from build123d import *

# Parameters (mm, degrees)
SKETCH2_R           = 2.35
BOSS_EXTRUDE1_DEPTH = 1.85
SKETCH3_R           = 2.35
BOSS_EXTRUDE2_DEPTH = 0.65
BOSS_EXTRUDE2_DRAFT = -45
SKETCH4_R           = 3
BOSS_EXTRUDE3_DEPTH = 6.5
CUT_EXTRUDE1_DEPTH  = 3
CHAMFER1_SIZE       = 0.6135


with BuildPart() as part:
    # Sketch1 → Revolve1 (revolve)
    with BuildSketch(Plane.XY, mode=Mode.PRIVATE) as revolve1_sk:
        with BuildLine():
            Line((-6, 6.5), (-6, 0))
            Line((-6, 0), (100, 0))
            Line((100, 0), (100, 4))
            Line((100, 4), (1, 4))
            Line((1, 4), (0.7, 3.7))
            ThreePointArc((0.7, 3.7), (0.201222236, 3.864777793), (0, 4.35))
            Line((0, 4.35), (0, 6.5))
            Line((0, 6.5), (-6, 6.5))
        make_face()
    revolve(revolve1_sk.sketch.rotate(Axis((-6, 0, 0), (1, 0, 0)), 270), axis=Axis((-6, 0, 0), (1, 0, 0)))

    # Sketch2 → Boss-Extrude1 (add)
    with BuildSketch(Plane(origin=(100, 0, 0), x_dir=(0, 0, -1), z_dir=(1, 0, 0))):
        with Locations(Location((0, 0, 0), (0, 0, 180))):
            Circle(SKETCH2_R)
    extrude(amount=BOSS_EXTRUDE1_DEPTH)


with BuildPart() as boss_extrude2_tool:
    # Sketch3 → Boss-Extrude2 (with draft: the straight prism first)
    with BuildSketch(Plane(origin=(101.85, 0, 0), x_dir=(0, 0, -1), z_dir=(1, 0, 0))):
        with Locations(Location((0, 0, 0), (0, 0, 180))):
            Circle(SKETCH3_R)
    extrude(amount=BOSS_EXTRUDE2_DEPTH)
    # Boss-Extrude2: the draft: its side faces are tilted about the plane it starts from
    boss_extrude2_sides = [boss_extrude2_tool.faces().sort_by_distance(p)[0] for p in [
        (102.175, 0, -2.35),
    ]]
    draft(boss_extrude2_sides, Plane(origin=(101.85, 0, 0), x_dir=(0, 0, -1), z_dir=(1, 0, 0)), BOSS_EXTRUDE2_DRAFT)


with BuildPart() as part_1:
    add(part.part)

    # Boss-Extrude2: add boss_extrude2_tool
    add(boss_extrude2_tool.part)

    # Sketch4 → Boss-Extrude3 (add)
    with BuildSketch(Plane(origin=(102.5, 0, 0), x_dir=(0, 0, -1), z_dir=(1, 0, 0))):
        Circle(SKETCH4_R)
    extrude(amount=BOSS_EXTRUDE3_DEPTH)

    # Sketch5 → Cut-Extrude1 (cut)
    with BuildSketch(Plane.ZY.offset(6)):
        Polygon((0, -2.886751346), (2.5, -1.443375673), (2.5, 1.443375673), (0, 2.886751346), (-2.5, 1.443375673), (-2.5, -1.443375673), align=None)
    extrude(amount=-CUT_EXTRUDE1_DEPTH, mode=Mode.SUBTRACT)

    # Sketch6 → Cut-Revolve1 (revolve, cut)
    with BuildSketch(Plane.XY, mode=Mode.PRIVATE) as cut_revolve1_sk:
        Polygon((-3, 2.5), (-3, 0), (-1.556624327, 0), align=None)
    revolve(cut_revolve1_sk.sketch.rotate(Axis((-3, 0, 0), (1, 0, 0)), 270), axis=Axis((-3, 0, 0), (1, 0, 0)), mode=Mode.SUBTRACT)

    # Chamfer1
    chamfer1_edges = [part_1.edges().sort_by_distance(p)[0] for p in [
        (109, 0, 3),
        (-6, 0, 6.5),
    ]]
    chamfer(chamfer1_edges, length=CHAMFER1_SIZE)


solid = part_1.part
Input: part model. Units: mm. Frame: model coordinates. A direction names the side the tool comes from. Coordinates: 2 decimals unless noted, no trailing zeros. Loops run counter-clockwise (first coordinate to the right, second up) from the corner with the lowest first, then second, coordinate; pieces in that order, holes last.
Q1. Material intervals for line 1 (X direction, y = 3, z = 0.75); line 2 (X direction, y = 5.25, z = 1.75); line 3 (Z direction, x = 31.5, y = -2.75), sorted ascending.
Q2. Cut plane A-A (x = 95.5). Output: boundary loops of the cut face in (y, z), then the cut area to 3 significant figures.
Q3. Set-up query: faces 1 (the face through (0, -4.24, -1.54)), 2 (the face through (109, 0, 0)), 3 (the face through (-5, 0, -2.5)), 4 (the face through (100, -2, 2)). Return all of +Z, -Z, +X, -X, +Y, -Y with unobstructed straight access to the full face (end or side cutting, diameter ignored); none if empty.
Q4. Draft query along Z for faces 5 (the face through (105, 0, 3)), 6 (the face through (-4.521, 2.175, -1.233)), 7 (the face through (-6, 0, -3)). Return one class per face: +Z half, -Z half, draft (parallel to the pull), parting line (faces both ways), or undercut.
Q5. Contact query for flat-ended pins moving along their axis: pin 1 (2 mm diameter, centred on x = 17, y = 1.5, fed in from +Z); pin 2 (5 mm diameter, centred on x = 33, z = -1, fed in from -Y); pin 3 (6 mm diameter, centred on y = 5, z = 4, fed in from +X). Output: stop coordinate, or through.
Working result:
1. line 1: x = -6 to 100
1. line 2: x = -6 to 0
1. line 3: z = -2.9 to 2.9
2. outline: circle Ø8 at (0, 0)
2. area: 50.3 mm2
3. face 1: +X
3. face 2: +Z, -Z, +X, +Y, -Y
3. face 3: -X
3. face 4: none
4. face 5: parting line
4. face 6: undercut
4. face 7: draft
5. pin 1: stops at z = 3.97
5. pin 2: stops at y = -4
5. pin 3: stops at x = 100
